Model file for the job. Use its own axes, mm. Coordinates: 2 decimals unless noted, no trailing zeros. Order: outer loops, then holes, each group sorted by start corner. A loop starts at its lowest first (then second) coordinate and runs counter-clockwise, first axis right, second up. Notation, with made-up numbers: M 7,66.5 L 40,66.5 A21 ccw 40,84.5 Z; hole C 30.25,62 d10. An arc over 180 degrees is marked long. Return JSON: item names as keys, results as strings.
Autodesk Inventor part; units mm, degrees
ref_plane "YZ Plane" through (0, 0, 0) normal (1, 0, 0) x (0, 1, 0)
ref_plane "XZ Plane" through (0, 0, 0) normal (0, 1, 0) x (-1, 0, 0)
ref_plane "XY Plane" through (0, 0, 0) normal (0, 0, 1) x (1, 0, 0)
sketch "스케치4" plane through (0, 0, 0) normal (0, 0, 1) x (1, 0, 0)
  line L0 (0, 0) -> (435, 0)
  line L1 (435, 0) -> (435, 345)
  line L2 (435, 345) -> (0, 345)
  line L3 (0, 0) -> (-1038.851, 0)
  line L4 (-1038.851, 0) -> (-1038.851, 600)
  line L5 (0, 0) -> (-352.5186, 0)
  line L6 (-352.5186, 820) -> (0, 820)
  line L7 (0, 820) -> (0, 345)
  line L8 (-1038.851, 600) -> (-352.5186, 820)
  dimension "d46" = 435
  dimension "d47" = 1473.851
  dimension "d48" = 345
  dimension "d49" = 475
  dimension "d50" = 435
  dimension "d53" = 787.5186
  dimension "d56" = 600
extrude "돌출3" add sketch "스케치4" along normal blind 10
properties part number "사이드 카울"
Item 1: Drop flat-ended pins along their axis: pin 1 Ø8 at (x, y) = (-202, 333.5) entering from -Z; pin 2 Ø1 at (x, z) = (236.5, 3) entering from +Y. Give the stop position or say it passes through.
Check result:
{"pin 1": "stops at z = 0", "pin 2": "stops at y = 345"}
Item 2: Saw through at B-B (y = 581.5). Write the cut outline in (x, z).
Check result:
{"outline": "M -1038.85,0 L 0,0 L 0,10 L -1038.85,10 Z"}
Item 3: Wall check: line 1 (X direction, y = 465, z = 7); line 2 (Y direction, x = 8, z = 6.75); line 3 (Y direction, x = -513.5, z = 5). Give the ranges that are in metal, low to high.
Check result:
{"line 1": "x = -1038.85 to 0", "line 2": "y = 0 to 345", "line 3": "y = 0 to 768.4"}
Item 4: Saw through at C-C (x = 341). Write the cut outline in (y, z).
Check result:
{"outline": "M 0,0 L 345,0 L 345,10 L 0,10 Z"}
Item 5: Saw through at A-A (z = 2.75). Write the cut outline in (x, y).
Check result:
{"outline": "M -1038.85,0 L 435,0 L 435,345 L 0,345 L 0,820 L -352.52,820 L -1038.85,600 Z"}
